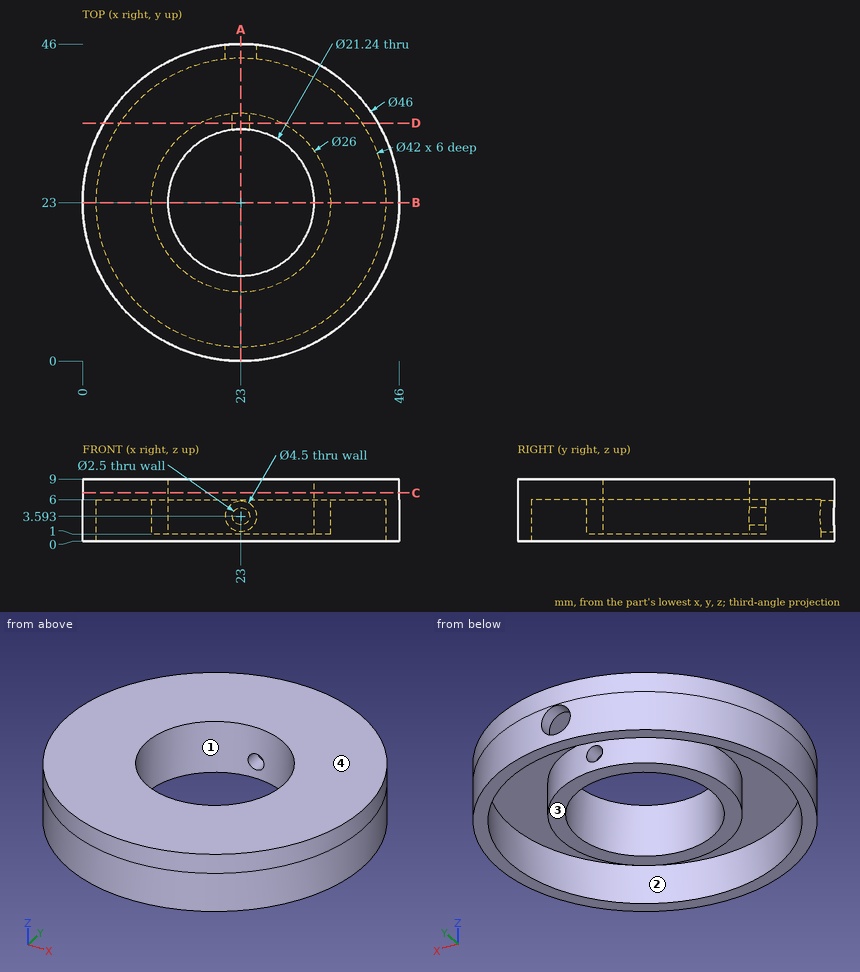
Design review of the part shown in the three views and the two pictorial views. Dimensions are in mm from the part's minimum x, y and z. A direction names the side the tool comes from. Round coordinates to 2 decimals unless told otherwise and drop trailing zeros. Write each loop counter-clockwise with the first axis right and the second up, starting at its lowest first coordinate (ties: lowest second). Pieces come first, ordered by that corner, then holes. Notation, with made-up numbers: (37.25, 11.25) - (87.25, 11.25) arc R8 ccw to (87.25, 23.25) - close; hole circle Ø2 at (17, -29). An arc over 180 degrees is marked (long way). Return JSON: item names as keys, results as strings. Group by question number.
Item 1: For probe 1 along Y at (x, z) = (23, 5.25); probe 2 along X at (y, z) = (16.5, 3.25); probe 3 along Y at (x, z) = (23, 6.25), list the stretches that pass through material, from the lowest coordinate up. Write a range as [from, to].
Item 2: We need section C-C on z = 7. Write out the cut boundary in (x, y).
Item 3: Insertion check: P1, Ø1.5, axis at x = 36, z = 2.5, coming from the +Y side; P2, Ø21, axis at x = 17, y = 16, coming from the -Z side; P3, Ø3, axis at x = 23, z = 3.59, coming from the +Y side. Each pin has a flat end and moves straight along its axis. Give the tip position at first contact, or say it passes through.
Item 4: We need section B-B on y = 23. Write out the cut boundary in (x, z).
Item 5: We need section A-A on x = 23. Write out the cut boundary in (y, z).
Item 6: Machinability: for the marked faces 1 and 2, which of the approach directions +Z, -Z, +X, -X, +Y, -Y give a long, thin tool a straight path to every point of the face, cutting with its end or side? Answer none if there is none.
Item 7: The part is to be moulded in two halves that separate along X. For the marked faces 3 and 4, say which applies: pulls with the +X half, pulls with the -X half, needs draft (parallel to the pull), parting line crosses it, or undercut.
Item 8: We need section D-D on y = 34.5. Write out the cut boundary in (x, z), and give its area (3 significant figures).
Model answer:
{
 "1": {"probe 1": "y = [0, 2], [10, 12.38], [33.62, 36]", "probe 2": "x = [0.94, 3.03], [11.74, 14.6], [31.4, 34.26], [42.97, 45.06]", "probe 3": "y = [0, 12.38], [33.62, 46]"},
 "2": {"outline": "circle Ø46 at (23, 23); hole circle Ø21.24 at (23, 23)"},
 "3": {"P1": "stops at y = 42.47", "P2": "stops at z = 1", "P3": "stops at y = 36"},
 "4": {"outline": "(0, 0) - (2, 0) - (2, 6) - (10, 6) - (10, 1) - (12.38, 1) - (12.38, 9) - (0, 9) - close; (33.62, 1) - (36, 1) - (36, 6) - (44, 6) - (44, 0) - (46, 0) - (46, 9) - (33.62, 9) - close"},
 "5": {"outline": "(0, 0) - (2, 0) - (2, 6) - (10, 6) - (10, 1) - (12.38, 1) - (12.38, 9) - (0, 9) - close; (33.62, 1) - (36, 1) - (36, 2.34) - (33.62, 2.34) - close; (33.62, 4.84) - (36, 4.84) - (36, 6) - (44, 6) - (44, 5.84) - (46, 5.84) - (46, 9) - (33.62, 9) - close; (44, 0) - (46, 0) - (46, 1.34) - (44, 1.34) - close"},
 "6": {"face 1": "+Z, -Z", "face 2": "-Z"},
 "7": {"face 3": "undercut", "face 4": "needs draft"},
 "8": {"outline": "(3.08, 0) - (5.43, 0) - (5.43, 6) - (16.94, 6) - (16.94, 1) - (29.06, 1) - (29.06, 6) - (40.57, 6) - (40.57, 0) - (42.92, 0) - (42.92, 9) - (3.08, 9) - close; hole circle Ø2.5 at (23, 3.59)", "area": "203 mm²"}
}
